```python
from build123d import *

# Parameters (mm, degrees)
BOSS_EXTRUDE1_DEPTH  = 5
BOSS_EXTRUDE7_DEPTH  = 5.75
BOSS_EXTRUDE8_START  = -3
BOSS_EXTRUDE8_DEPTH  = 3
SKETCH15_R           = 2.75
CUT_EXTRUDE7_DEPTH   = 46.783095044
FILLET2_R            = 5
SKETCH16_W           = 12
SKETCH16_H           = 3
CUT_EXTRUDE8_DEPTH   = 23
SKETCH17_R           = 2.35
CUT_EXTRUDE9_DEPTH   = 32
CUT_EXTRUDE11_START  = -8
CUT_EXTRUDE11_DEPTH  = 3.8
LPATTERN1_COUNT      = 2
LPATTERN1_PITCH      = 10
SKETCH26_R           = 11
CUT_EXTRUDE12_DEPTH  = 7.5
SKETCH28_W           = 29.000715486
SKETCH28_H           = 0.6
SKETCH28_W_2         = 23
SKETCH28_W_3         = 27.103937603
SKETCH28_W_4         = 25.207159719
BOSS_EXTRUDE9_DEPTH  = 3
BOSS_EXTRUDE10_DEPTH = 0.4


with BuildPart() as part:
    # Sketch1 → Boss-Extrude1 (new body)
    with BuildSketch(Plane.XY):
        with BuildLine():
            Line((-40.155138696, -0.836255417), (-17.155138696, -0.836255417))
            Line((-17.155138696, -0.836255417), (-5.547811002, -9.922989015))
            ThreePointArc((-5.547811002, -9.922989015), (7.086733598, -8.384066419), (5.547811002, 4.250478181))
            Line((5.547811002, 4.250478181), (-10.947501986, 17.163744583))
            Line((-10.947501986, 17.163744583), (-40.155138696, 17.163744583))
            Line((-40.155138696, 17.163744583), (-40.155138696, -0.836255417))
        make_face()
    extrude(amount=BOSS_EXTRUDE1_DEPTH)

    # Sketch14 → Boss-Extrude7 (add)
    with BuildSketch(Plane.XY.offset(5)):
        with BuildLine():
            Line((-40.155138696, -0.836255417), (-40.155138696, 17.163744583))
            Line((-40.155138696, 17.163744583), (-10.947501986, 17.163744583))
            Line((-10.947501986, 17.163744583), (5.547811002, 4.250478181))
            ThreePointArc((5.547811002, 4.250478181), (7.086733598, -8.384066419), (-5.547811002, -9.922989015))
            Line((-5.547811002, -9.922989015), (-17.155138696, -0.836255417))
            Line((-17.155138696, -0.836255417), (-40.155138696, -0.836255417))
        make_face()
    extrude(amount=BOSS_EXTRUDE7_DEPTH)

    # Sketch27 → Boss-Extrude8 (add)
    with BuildSketch(Plane.XY.offset(BOSS_EXTRUDE8_START)):
        with BuildLine():
            Line((-17.155138696, -0.836255417), (-10.947501986, 17.163744583))
            Line((-10.947501986, 17.163744583), (5.547811002, 4.250478181))
            ThreePointArc((5.547811002, 4.250478181), (7.086733598, -8.384066419), (-5.547811002, -9.922989015))
            Line((-5.547811002, -9.922989015), (-17.155138696, -0.836255417))
        make_face()
    extrude(amount=BOSS_EXTRUDE8_DEPTH)

    # Sketch15 → Cut-Extrude7 (cut, through all)
    with BuildSketch(Plane(origin=(0, 0, -3), x_dir=(-1, 0, 0), z_dir=(0, 0, -1))):
        with Locations((0, -2.836255417)):
            Circle(SKETCH15_R)
    extrude(amount=-CUT_EXTRUDE7_DEPTH, mode=Mode.SUBTRACT)

    # Fillet2
    # the kernel refuses this fillet: 5 mm, written as the material it takes off along each edge
    with BuildSketch(Plane(origin=(-20.89022917, -11.666726282, -3), x_dir=(0.9453610009462032, -0.32602542522016986, 0), z_dir=(0.3260254252201699, 0.9453610009462033, 0))) as fillet2_piece_1:
        with BuildLine():
            CenterArc((4.582575695, -5), FILLET2_R, 90, 66.421821522)
            Line((0, -3), (-0.091651514, -2.96))
            ThreePointArc((-0.091651514, -2.96), (-0.1, -1.5), (-0.1, 0))
            Line((-0.1, 0), (0, 0.1))
            Line((0, 0.1), (4.582575695, 0.1))
            Line((4.582575695, 0.1), (4.582575695, 0))
        make_face()
    extrude(amount=41.95322389, mode=Mode.SUBTRACT)

    # Mirror1: part across plane


with BuildPart() as part_1:
    add(part.part)
    add(part.part.mirror(Plane(origin=(0, -2.836255417, 10.75), x_dir=(1, 0, 0), z_dir=(0, 0, 1))))

    # Sketch16 → Cut-Extrude8 (cut)
    with BuildSketch(Plane.ZY.offset(40.155138696)):
        with Locations((10.75, 0.663744583)):
            Rectangle(SKETCH16_W, SKETCH16_H)
        with Locations((10.75, 15.663744583)):
            Rectangle(SKETCH16_W, SKETCH16_H)
    extrude(amount=-CUT_EXTRUDE8_DEPTH, mode=Mode.SUBTRACT)

    # Sketch17 → Cut-Extrude9 (cut)
    with BuildSketch(Plane.ZY.offset(40.155138696)):
        with Locations((10.75, 8.163744583)):
            Circle(SKETCH17_R)
    extrude(amount=-CUT_EXTRUDE9_DEPTH, mode=Mode.SUBTRACT)

    # Sketch20 → Cut-Extrude11 (cut)
    with BuildSketch(Plane.ZY.offset(40.155138696).offset(CUT_EXTRUDE11_START)):
        Polygon((14.5, 2.163744583), (14.5, 5.998681073), (10.75, 3.833617564), (7, 5.998681073), (7, 2.163744583), align=None)
        Polygon((10.75, 3.833617564), (14.5, 5.998681073), (14.5, 10.328808092), (10.75, 12.493871602), (7, 10.328808092), (7, 5.998681073), align=None)
    cut_extrude11 = extrude(amount=-CUT_EXTRUDE11_DEPTH, mode=Mode.SUBTRACT)

    # LPattern1: Cut-Extrude11 ×2
    with Locations(*[(i * LPATTERN1_PITCH, 0, 0) for i in range(1, LPATTERN1_COUNT)]):
        add(cut_extrude11, mode=Mode.SUBTRACT)

    # Sketch26 → Cut-Extrude12 (cut, symmetric)
    with BuildSketch(Plane.XY.offset(10.75)):
        with Locations((0, -2.836255417)):
            Circle(SKETCH26_R)
    extrude(amount=CUT_EXTRUDE12_DEPTH, both=True, mode=Mode.SUBTRACT)

    # Sketch28 → Boss-Extrude9 (add)
    with BuildSketch(Plane(origin=(0, 0, -3), x_dir=(-1, 0, 0), z_dir=(0, 0, -1))):
        with Locations((25.654780953, 16.863744583)):
            Rectangle(SKETCH28_W, SKETCH28_H)
        with Locations((28.655138696, -0.536255417)):
            Rectangle(SKETCH28_W_2, SKETCH28_H)
        with Locations((26.603169895, 11.363744583)):
            Rectangle(SKETCH28_W_3, SKETCH28_H)
        with Locations((27.551558836, 5.863744583)):
            Rectangle(SKETCH28_W_4, SKETCH28_H)
    extrude(amount=-BOSS_EXTRUDE9_DEPTH)

    # Sketch29 → Boss-Extrude10 (add)
    with BuildSketch(Plane(origin=(0, 0, -3), x_dir=(-1, 0, 0), z_dir=(0, 0, -1))):
        Polygon((40.155138696, 17.163744583), (40.155138696, -0.836255417), (17.155138696, -0.836255417), (11.15442321, 16.563744583), (10.947501986, 17.163744583), align=None)
    extrude(amount=-BOSS_EXTRUDE10_DEPTH)


solid = part_1.part
```
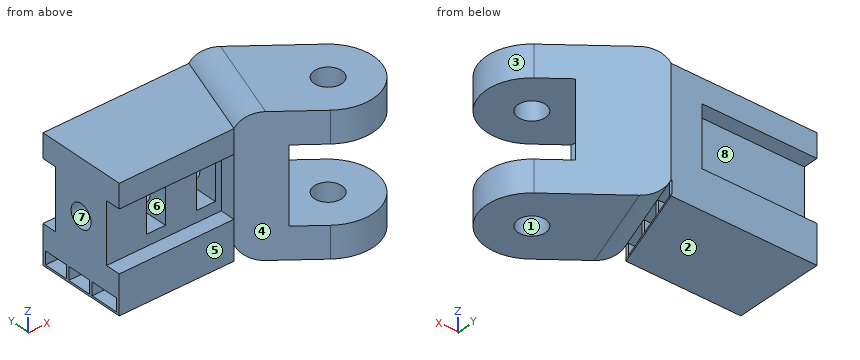
Could you check a few things on this model? Use its own coordinates, in mm. Face numbers are marked on the shaded views. A direction names the side the tool comes from. Coordinates: 2 decimals unless noted, no trailing zeros. Write each loop counter-clockwise with the first axis right and the second up, starting at its lowest first coordinate (ties: lowest second). Pieces come first, ordered by that corner, then holes. Notation, with made-up numbers: (71, 18) - (103, 18) arc R35 cw to (103, 53) - close; hole circle Ø6 at (57.25, 36.5). An arc over 180 degrees is marked (long way). Use a Markdown table: item, result.
Q1. Imagine slicing it at D-D (z = 2.5). List the corners of the cut face in (x, y) for me, and give its area (3 significant figures).
Geometry check:
| item | result |
|---|---|
| outline | (-40.16, -0.84) - (-17.16, -0.84) - (-5.55, -9.92) arc R9 ccw to (5.55, 4.25) - (-10.95, 17.16) - (-40.16, 17.16) - close; hole circle Ø5.5 at (0, -2.84) |
| area | 895 mm2 |
Q2. I'm going to push flat-ended pins straight in: pin 1 Ø4 at (y, z) = (8.16, 10.75) entering from -X; pin 2 Ø0.7 at (y, z) = (17, -1) entering from +X; pin 3 Ø6 at (x, y) = (-23, 14.5) entering from +Z. Where does each tip first touch, or does it pass through?
Geometry check:
| item | result |
|---|---|
| pin 1 | stops at x = -8.16 |
| pin 2 | stops at x = -10.29 |
| pin 3 | stops at z = 21.5 |
Q3. Imagine slicing it at B-B (x = -0.5). List the corners of the cut face in (y, z) for me, and give its area (3 significant figures).
Geometry check:
| item | result |
|---|---|
| outline | (-11.82, -3) - (-5.54, -3) - (-5.54, 3.25) - (-11.82, 3.25) - close; (-11.82, 18.25) - (-5.54, 18.25) - (-5.54, 24.5) - (-11.82, 24.5) - close; (-0.13, -3) - (8.98, -3) - (8.98, 24.5) - (-0.13, 24.5) - (-0.13, 18.25) - (8.15, 18.25) - (8.15, 3.25) - (-0.13, 3.25) - close |
| area | 205 mm2 |
Q4. Thinking about a two-plate mould opening in X: for the marked faces 1, 2, 3 and 4, which applies, +X half, -X half, draft (parallel to the pull), parting line (faces both ways), or undercut?
Geometry check:
| item | result |
|---|---|
| face 1 | undercut |
| face 2 | draft |
| face 3 | parting line |
| face 4 | -X half |
Q5. Which directions (+Z, -Z, +X, -X, +Y, -Y) give clear straight access to the entire face, cutting with the end or side of a thin tool? Please do the marked faces 5, 6, 7 and 8.
Geometry check:
| item | result |
|---|---|
| face 5 | +Z, -Z, -X, -Y |
| face 6 | -Y |
| face 7 | -X |
| face 8 | -X, +Y |
Q6. Imagine slicing it at A-A (x = -19.5). Count the separate pieces of the cut face and the enclosed holes in it, and give its area (3 significant figures).
Geometry check:
| item | result |
|---|---|
| separate pieces | 1 |
| enclosed holes | 3 |
| area | 259 mm2 |
Q7. Please list where these lines run through material, in increasing order: L1, parallel to Z at x = -33.5, y = 12.5; L2, parallel to Z at x = -26, y = 1.5; L3, parallel to Y at x = -37, z = 10.75.
Geometry check:
| item | result |
|---|---|
| L1 | z = -3 to -2.6, 0 to 21.5 |
| L2 | z = -3 to -2.6, 0 to 4.75, 16.75 to 21.5 |
| L3 | y = 2.16 to 5.81, 10.51 to 14.16 |
